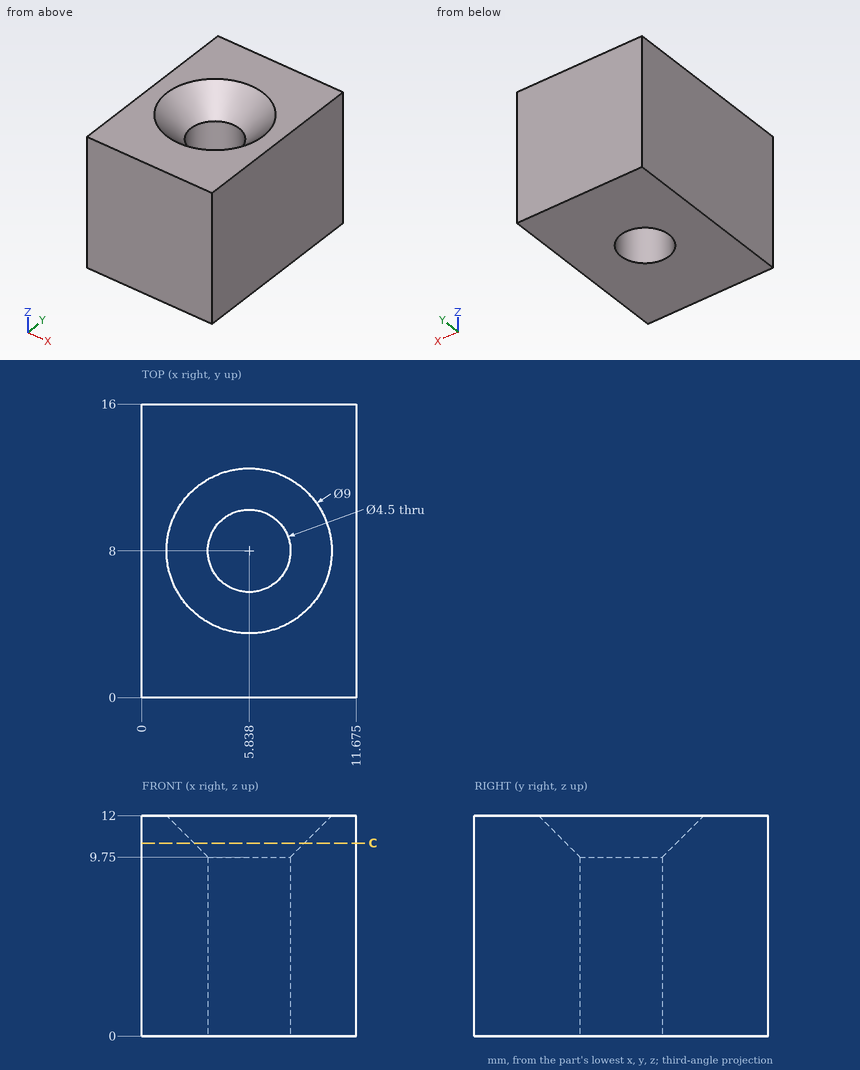
Print and shaded views of the part. All mm, measured from the part's lowest x, y and z. Coordinates: 2 decimals unless noted, no trailing zeros. Loops run counter-clockwise (first coordinate to the right, second up) from the corner with the lowest first, then second, coordinate; pieces in that order, holes last. Notation, with made-up numbers: (47, -3.5) - (58, -3.5) arc R4 ccw to (58, 2.5) - close; hole circle Ø2 at (42.5, 71.25). An arc over 180 degrees is marked (long way). Write item = value, one per line. Start each with the question number.
Item 1: Drop flat-ended pins along their axis: pin 1 Ø3 at (x, y) = (7.5, 10) entering from +Z; pin 2 Ø6 at (x, y) = (5.84, 8) entering from +Z. Give the stop position or say it passes through.
Item 2: Saw through at C-C, the plane z = 10.5. List the corners of the cut face in (x, y) (1 decimal).
Item 3: Wall check: probe 1 along X at (y, z) = (8, 6.25) (1 decimal); probe 2 along Y at (x, z) = (6, 5.5) (1 decimal); probe 3 along X at (y, z) = (8.75, 8.75) (1 decimal). Give the ranges that are in metal, low to high. Write a range as [from, to].
Answers:
q1.pin_1 = 11.6
q1.pin_2 = 10.5
q2.outline = (0, 0) - (11.7, 0) - (11.7, 16) - (0, 16) - close; hole circle Ø6 at (5.8, 8)
q3.probe_1 = [0, 3.6], [8.1, 11.7]
q3.probe_2 = [0, 5.8], [10.2, 16]
q3.probe_3 = [0, 3.7], [8, 11.7]
